Design review of the part built by this model. Coordinates are the model's own, in mm. Give positions to 0.01 mm unless a question says otherwise; leave off trailing zeros. Loops run counter-clockwise (first coordinate to the right, second up) from the corner with the lowest first, then second, coordinate; pieces in that order, holes last.
from build123d import *

# Parameters (mm, degrees)
F0_R     = 3
F0_W     = 45.8
F0_H     = 36
F1_DEPTH = 2


with BuildPart() as f1:
    # F0 (on Top) → F1 (new body)
    with BuildSketch(Plane.XY):
        with BuildLine():
            Line((-100.743165, 71.169704), (-100.743165, 74.341277))
            ThreePointArc((-100.743165, 74.341277), (-130.743165, -0.658723), (-100.743165, -75.658723))
            Line((-100.743165, -75.658723), (-100.743165, -32.48715))
            ThreePointArc((-100.743165, -32.48715), (-102.743165, -29.658723), (-100.743165, -26.830296))
            Line((-100.743165, -26.830296), (-100.743165, -15.658723))
            Line((-100.743165, -15.658723), (-107.243165, -15.658723))
            Line((-107.243165, -15.658723), (-107.243165, 19.341277))
            Line((-107.243165, 19.341277), (-107.243165, 54.341277))
            Line((-107.243165, 54.341277), (-100.743165, 54.341277))
            Line((-100.743165, 54.341277), (-100.743165, 65.51285))
            ThreePointArc((-100.743165, 65.51285), (-102.743165, 68.341277), (-100.743165, 71.169704))
        make_face()
        with Locations((-113.993165, -9.158723)):
            Circle(F0_R, mode=Mode.SUBTRACT)
        with Locations((-113.993165, 47.841277)):
            Circle(F0_R, mode=Mode.SUBTRACT)
        with BuildLine():
            Line((-10.743165, 74.341277), (-100.743165, 74.341277))
            Line((-100.743165, 74.341277), (-100.743165, 71.169704))
            ThreePointArc((-100.743165, 71.169704), (-98.011114, 70.790767), (-96.743165, 68.341277))
            ThreePointArc((-96.743165, 68.341277), (-98.011114, 65.891788), (-100.743165, 65.51285))
            Line((-100.743165, 65.51285), (-100.743165, 54.341277))
            Line((-100.743165, 54.341277), (-67.243165, 54.341277))
            Line((-67.243165, 54.341277), (-67.243165, 19.341277))
            Line((-67.243165, 19.341277), (-67.243165, -15.658723))
            Line((-67.243165, -15.658723), (-100.743165, -15.658723))
            Line((-100.743165, -15.658723), (-100.743165, -26.830296))
            ThreePointArc((-100.743165, -26.830296), (-98.011114, -27.209233), (-96.743165, -29.658723))
            ThreePointArc((-96.743165, -29.658723), (-98.011114, -32.108212), (-100.743165, -32.48715))
            Line((-100.743165, -32.48715), (-100.743165, -75.658723))
            Line((-100.743165, -75.658723), (-50.743165, -75.658723))
            Line((-50.743165, -75.658723), (-50.743165, -35.658723))
            Line((-50.743165, -35.658723), (-10.743165, -35.658723))
            Line((-10.743165, -35.658723), (-10.743165, 74.341277))
        make_face()
        with Locations((-60.743165, -13.158723)):
            Circle(F0_R, mode=Mode.SUBTRACT)
        with Locations((-38.343165, 19.341277)):
            Rectangle(F0_W, F0_H, mode=Mode.SUBTRACT)
        with Locations((-60.743165, 51.841277)):
            Circle(F0_R, mode=Mode.SUBTRACT)
        with BuildLine():
            Line((79.256835, 74.341277), (-10.743165, 74.341277))
            Line((-10.743165, 74.341277), (-10.743165, -35.658723))
            Line((-10.743165, -35.658723), (34.256835, -35.658723))
            Line((34.256835, -35.658723), (34.256835, -75.658723))
            Line((34.256835, -75.658723), (79.256835, -75.658723))
            Line((79.256835, -75.658723), (79.256835, -32.48715))
            ThreePointArc((79.256835, -32.48715), (75.256835, -29.658723), (79.256835, -26.830296))
            Line((79.256835, -26.830296), (79.256835, -15.658723))
            Line((79.256835, -15.658723), (45.756835, -15.658723))
            Line((45.756835, -15.658723), (45.756835, 19.341277))
            Line((45.756835, 19.341277), (45.756835, 54.341277))
            Line((45.756835, 54.341277), (79.256835, 54.341277))
            Line((79.256835, 54.341277), (79.256835, 65.51285))
            ThreePointArc((79.256835, 65.51285), (75.256835, 68.341277), (79.256835, 71.169704))
            Line((79.256835, 71.169704), (79.256835, 74.341277))
        make_face()
        with Locations((39.256835, -13.158723)):
            Circle(F0_R, mode=Mode.SUBTRACT)
        with Locations((16.856835, 19.341277)):
            Rectangle(F0_W, F0_H, mode=Mode.SUBTRACT)
        with Locations((39.256835, 51.841277)):
            Circle(F0_R, mode=Mode.SUBTRACT)
        with BuildLine():
            ThreePointArc((79.256835, -75.658723), (109.256835, -0.658723), (79.256835, 74.341277))
            Line((79.256835, 74.341277), (79.256835, 71.169704))
            ThreePointArc((79.256835, 71.169704), (80.706325, 70.073328), (81.256835, 68.341277))
            ThreePointArc((81.256835, 68.341277), (80.706325, 66.609227), (79.256835, 65.51285))
            Line((79.256835, 65.51285), (79.256835, 54.341277))
            Line((79.256835, 54.341277), (85.756835, 54.341277))
            Line((85.756835, 54.341277), (85.756835, 19.341277))
            Line((85.756835, 19.341277), (85.756835, -15.658723))
            Line((85.756835, -15.658723), (79.256835, -15.658723))
            Line((79.256835, -15.658723), (79.256835, -26.830296))
            ThreePointArc((79.256835, -26.830296), (80.706325, -27.926672), (81.256835, -29.658723))
            ThreePointArc((81.256835, -29.658723), (80.706325, -31.390773), (79.256835, -32.48715))
            Line((79.256835, -32.48715), (79.256835, -75.658723))
        make_face()
        with Locations((92.506835, -9.158723)):
            Circle(F0_R, mode=Mode.SUBTRACT)
        with Locations((92.506835, 47.841277)):
            Circle(F0_R, mode=Mode.SUBTRACT)
    extrude(amount=F1_DEPTH)


solid = f1.part
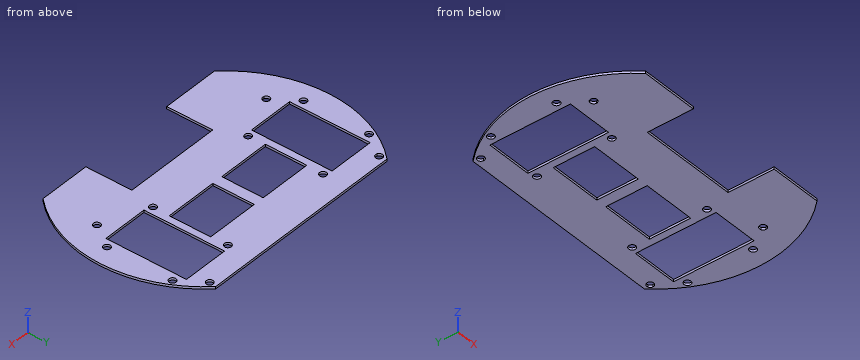
Q1. Take a section at D-D (z = 0.7). Give the number of separate pieces and of enclosed holes in the cut face, plus the area to 3 significant figures.
Results:
separate pieces: 1
enclosed holes: 16
area: 20,600 mm2
Q2. Take a section at B-B (y = 11.5). Give the boundary of the cut face in (x, z) (3 decimals).
Results:
outline: (-130.061, 0) - (-107.243, 0) - (-107.243, 2) - (-130.061, 2) - close; (-67.243, 0) - (-61.243, 0) - (-61.243, 2) - (-67.243, 2) - close; (-15.443, 0) - (-6.043, 0) - (-6.043, 2) - (-15.443, 2) - close; (39.757, 0) - (45.757, 0) - (45.757, 2) - (39.757, 2) - close; (85.757, 0) - (108.575, 0) - (108.575, 2) - (85.757, 2) - close
Q3. Take a section at A-A (x = 71.5). Give the boundary of the cut face in (y, z), plus the area to 3 significant figures.
Results:
outline: (-75.66, 0) - (-15.66, 0) - (-15.66, 2) - (-75.66, 2) - close; (54.34, 0) - (74.34, 0) - (74.34, 2) - (54.34, 2) - close
area: 160 mm2
Q4. Wall thickness on line 1 (Y direction, x = -61, z = 0.75); line 2 (Y direction, x = 58, z = 1.65); line 3 (Y direction, x = 78.5, z = 0.7): over which ranges is each line inside the solid? List them lowest first.
Results:
line 1: y = -75.66 to -16.15, -10.17 to 1.34, 37.34 to 48.85, 54.83 to 74.34
line 2: y = -75.66 to -15.66, 54.34 to 74.34
line 3: y = -75.66 to -32.65, -26.67 to -15.66, 54.34 to 65.35, 71.33 to 74.34
Q5. Take a section at C-C (y = -46.5). Give the boundary of the cut face in (x, z), plus the area to 3 significant figures.
Results:
outline: (-120.61, 0) - (-50.74, 0) - (-50.74, 2) - (-120.61, 2) - close; (34.26, 0) - (99.12, 0) - (99.12, 2) - (34.26, 2) - close
area: 269 mm2
Q6. Insertion check: pin 1 (1 mm diameter, centred on y = 12.5, z = 0.5, fed in from +X); pin 2 (1 mm diameter, centred on y = -8.5, z = 1, fed in from -X); pin 3 (0.6 mm diameter, centred on x = -11, z = 1, fed in from -Y). Each pin has a flat end and moves straight along its axis. Give the tip position at first contact, or say it passes through.
Results:
pin 1: stops at x = 108.52
pin 2: stops at x = -130.5
pin 3: stops at y = -35.66
